The model under review builds one solid part; all positions refer to its coordinate system, in mm. Face numbers are marked on the shaded views. A direction names the side the tool comes from. Round coordinates to 2 decimals unless told otherwise and drop trailing zeros. Order: outer loops, then holes, each group sorted by start corner. A loop starts at its lowest first (then second) coordinate and runs counter-clockwise, first axis right, second up. Notation, with made-up numbers: M 30,-29 L 89,-29 A21 cw 89,-1 Z; hole C 38.5,2 d4. An arc over 180 degrees is marked long. Answer as a JSON object with one key per item and string values. Group by question number.
1. Add section A-A on z = 0. State the section outline as (x, y) points.
2. Add section C-C on y = 2.1. State the section outline as (x, z) points, and give its area (3 significant figures).
3. Clearance check with flat-ended pins moving along their axes: P1, Ø1.6, axis at x = -15.5, y = 0, coming from the +Z side; P2, Ø0.6, axis at x = -16, y = 0.5, coming from the -Z side; P3, Ø8.5, axis at x = 0, z = 0, coming from the +Y side; P4, Ø5, axis at x = 5.5, z = -6.5, coming from the +Y side. State where each tip first meets the part, or that it passes through.
4. To check wall thickness, follow probe 1 along Y at (x, z) = (-18.5, -6.25); probe 2 along X at (y, z) = (0.2, 0); probe 3 along Z at (x, y) = (-12.5, -0.2). State the ranges of each line that lie inside material, in increasing order. Write a range as [from, to].
5. Add section D-D on y = -1.55. State the section outline as (x, z) points, and give its area (3 significant figures).
6. Add section B-B on x = -10. State the section outline as (y, z) points, and give its area (3 significant figures).
7. Machinability: for the marked faces 1 and 2, which of the approach directions +Z, -Z, +X, -X, +Y, -Y give a long, thin tool a straight path to every point of the face, cutting with its end or side? Answer none if there is none.
8. Mouldability with a two-part tool opening along X and no side actions: class the marked faces 3, 4 and 5 as released by +X, released by -X, zero draft, split by the parting line, or undercut.
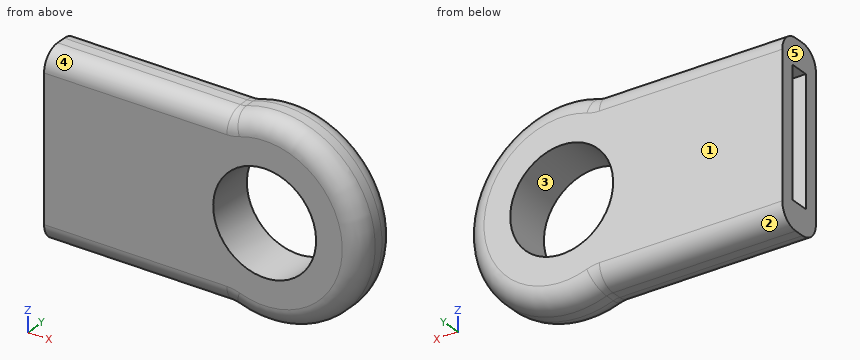
```python
from build123d import *

# Parameters (mm, degrees)
CROQUIS1_R              = 5.3
SALIENTE_EXTRUIR1_DEPTH = 2.5
CROQUIS2_W              = 13.1
CROQUIS2_H              = 2
CORTAR_EXTRUIR1_DEPTH   = 15
REDONDEO1_R             = 2


with BuildPart() as part:
    # Croquis1 → Saliente-Extruir1 (new, symmetric)
    with BuildSketch(Plane(origin=(0, 0, 0), x_dir=(1, 0, 0), z_dir=(0, 1, 0))):
        with BuildLine():
            Line((-22.725121358, 9.35), (-3.546477125, 9.35))
            ThreePointArc((-3.546477125, 9.35), (10, 0), (-3.546477125, -9.35))
            Line((-3.546477125, -9.35), (-22.725121358, -9.35))
            Line((-22.725121358, -9.35), (-22.725121358, 9.35))
        make_face()
        with Locations(Location((0, 0, 0), (0, 0, 270))):
            Circle(CROQUIS1_R, mode=Mode.SUBTRACT)
    extrude(amount=SALIENTE_EXTRUIR1_DEPTH, both=True)

    # Croquis2 → Cortar-Extruir1 (cut)
    with BuildSketch(Plane.ZY.offset(22.725121358)):
        Rectangle(CROQUIS2_W, CROQUIS2_H)
    extrude(amount=-CORTAR_EXTRUIR1_DEPTH, mode=Mode.SUBTRACT)

    # Redondeo1
    redondeo1_edges = [part.edges().sort_by_distance(p)[0] for p in [
        (10, 2.5, 0),
        (-13.135799242, 2.5, -9.35),
        (-13.135799242, -2.5, -9.35),
        (10, -2.5, 0),
        (-13.135799242, -2.5, 9.35),
        (-13.135799242, 2.5, 9.35),
        (-3.546477125, 0, -9.35),
        (-3.546477125, 0, 9.35),
    ]]
    fillet(redondeo1_edges, radius=REDONDEO1_R)


solid = part.part
```
Recorded:
{
 "1": {"outline": "M -22.73,-2.5 L -5.3,-2.5 L -5.3,2.5 L -22.73,2.5 L -22.73,1 L -7.73,1 L -7.73,-1 L -22.73,-1 Z; M 5.3,-2.5 L 8,-2.5 A2 ccw 10,-0.5 L 10,0.5 A2 ccw 8,2.5 L 5.3,2.5 Z"},
 "2": {"outline": "M -22.73,-8.55 L -3.9,-8.55 A2.8 cw -2.99,-8.7 A9.2 ccw long -2.99,8.7 A2.8 cw -3.9,8.55 L -22.73,8.55 Z; hole C 0,0 d10.6", "area": "436 mm²"},
 "3": {"P1": "stops at z = 9.35", "P2": "stops at z = -9.35", "P3": "passes through", "P4": "stops at y = 2.5"},
 "4": {"probe 1": "y = [-2.5, -1], [1, 2.5]", "probe 2": "x = [-7.73, -5.3], [5.3, 10]", "probe 3": "z = [-9.35, -6.55], [6.55, 9.35]"},
 "5": {"outline": "M -22.73,-9.05 L -3.9,-9.05 A2.3 cw -3.15,-9.18 A9.7 ccw long -3.15,9.18 A2.3 cw -3.9,9.05 L -22.73,9.05 Z; hole C 0,0 d10.6", "area": "474 mm²"},
 "6": {"outline": "M -2.5,-7.35 A2 ccw -0.5,-9.35 L 0.5,-9.35 A2 ccw 2.5,-7.35 L 2.5,7.35 A2 ccw 0.5,9.35 L -0.5,9.35 A2 ccw -2.5,7.35 Z; hole M -1,-6.55 L 1,-6.55 L 1,6.55 L -1,6.55 Z", "area": "63.9 mm²"},
 "7": {"face 1": "+Z, -Z, +X, -X, +Y", "face 2": "-Z, -X, +Y"},
 "8": {"face 3": "undercut", "face 4": "zero draft", "face 5": "released by -X"}
}
